Geometry check sheet. Reference: the model listing, model coordinates, mm. A direction names the side the tool comes from. Coordinates: 2 decimals unless noted, no trailing zeros. Write each loop counter-clockwise with the first axis right and the second up, starting at its lowest first coordinate (ties: lowest second). Pieces come first, ordered by that corner, then holes. Notation, with made-up numbers: (25, 51) -> (63, 51) arc R19 cw to (63, 61) -> close; hole circle Ø6 at (-5.75, -10). An arc over 180 degrees is marked (long way). Answer in a Markdown table with one row per item. Add a question column.
Q1. Thickness scan on line 1 (Y direction, x = 5, z = 1.7); line 2 (X direction, y = 10.5, z = 3); line 3 (Y direction, x = 5.5, z = 2.6). Record the ranges inside material, lowest first.
Q2. Section check A-A, the plane y = 10.5. Record the boundary of the cut face in (x, z), and give its area (3 significant figures).
Q3. Gauge pin test, flat ends, axial feed: P1, Ø1.2, axis at y = 7.5, z = 2, coming from the +X side; P2, Ø1.2, axis at x = -3, z = 2, coming from the -Y side. Record the tip position at first contact, or that the pin passes through.
Q4. Section check B-B, the plane x = 5. Record the boundary of the cut face in (y, z), and give its area (3 significant figures).
Q5. Release check for a two-part mould opening along Y. For faces 4 (the face through (5.211, 26.598, 1.972)), 5 (the face through (4.583, 24.094, 1.972)), 6 (the face through (7, 13.5, 4)) record: pulls with the +Y half, pulls with the -Y half, needs draft (parallel to the pull), parting line crosses it, or undercut.
Q6. Tool access check on faces 1 (the face through (0, 6, 2)), 2 (the face through (12, 12, 2)), 3 (the face through (-4.6, 15, 2)). Record the directions out of +Z, -Z, +X, -X, +Y, -Y that give a thin tool (end or side, any length) a straight path to the whole face; none if there is none.
Q7. Section check C-C, the plane z = 1.05. Record the boundary of the cut face in (x, y).
Q8. Section check D-D, the plane y = 6. Record the boundary of the cut face in (x, z).
```python
from build123d import *

# Parameters (mm, degrees)
BOSS_EXTRUDE1_DEPTH = 4
SKETCH2_W           = 2.5
SKETCH2_H           = 4
CUT_EXTRUDE1_DEPTH  = 4
SKETCH3_R           = 3.2
CUT_EXTRUDE2_DEPTH  = 5


with BuildPart() as part:
    # Sketch1 → Boss-Extrude1 (new body)
    with BuildSketch(Plane.XY):
        with BuildLine():
            Line((0, 0), (10, 0))
            Line((10, 0), (10, 4))
            Line((10, 4), (12.5, 4))
            Line((12.5, 4), (12.5, 8))
            Line((12.5, 8), (10, 8))
            Line((10, 8), (10, 12))
            Line((10, 12), (14.6, 12))
            Line((14.6, 12), (14.6, 17))
            ThreePointArc((14.6, 17), (5, 26.6), (-4.6, 17))
            Line((-4.6, 17), (-4.6, 12))
            Line((-4.6, 12), (0, 12))
            Line((0, 12), (0, 8))
            Line((0, 8), (-2.5, 8))
            Line((-2.5, 8), (-2.5, 4))
            Line((-2.5, 4), (0, 4))
            Line((0, 4), (0, 0))
        make_face()
    extrude(amount=BOSS_EXTRUDE1_DEPTH)

    # Sketch2 → Cut-Extrude1 (cut)
    with BuildSketch(Plane.XY.offset(4)):
        with Locations((-1.25, 6)):
            Rectangle(SKETCH2_W, SKETCH2_H)
        with Locations((11.25, 6)):
            Rectangle(SKETCH2_W, SKETCH2_H)
    extrude(amount=-CUT_EXTRUDE1_DEPTH, mode=Mode.SUBTRACT)

    # Sketch3 → Cut-Extrude2 (cut, through all)
    with BuildSketch(Plane.XY):
        with Locations((5, 20.921172359)):
            Circle(SKETCH3_R)
        with Locations((5, 10.5)):
            Circle(SKETCH3_R)
    extrude(amount=CUT_EXTRUDE2_DEPTH, mode=Mode.SUBTRACT)


solid = part.part
```
Calculated:
| question | item | result |
|---|---|---|
| 1 | line 1 | y = 0 to 7.3, 13.7 to 17.72, 24.12 to 26.6 |
| 1 | line 2 | x = 0 to 1.8, 8.2 to 10 |
| 1 | line 3 | y = 0 to 7.34, 13.66 to 17.76, 24.08 to 26.59 |
| 2 | outline | (0, 0) -> (1.8, 0) -> (1.8, 4) -> (0, 4) -> close; (8.2, 0) -> (10, 0) -> (10, 4) -> (8.2, 4) -> close |
| 2 | area | 14.4 mm² |
| 3 | P1 | stops at x = 10 |
| 3 | P2 | stops at y = 12 |
| 4 | outline | (0, 0) -> (7.3, 0) -> (7.3, 4) -> (0, 4) -> close; (13.7, 0) -> (17.72, 0) -> (17.72, 4) -> (13.7, 4) -> close; (24.12, 0) -> (26.6, 0) -> (26.6, 4) -> (24.12, 4) -> close |
| 4 | area | 55.2 mm² |
| 5 | face 4 | pulls with the +Y half |
| 5 | face 5 | undercut |
| 5 | face 6 | needs draft |
| 6 | face 1 | +Z, -Z, -X, -Y |
| 6 | face 2 | +Z, -Z, +X, -Y |
| 6 | face 3 | +Z, -Z, -X, +Y, -Y |
| 7 | outline | (-4.6, 12) -> (0, 12) -> (0, 0) -> (10, 0) -> (10, 12) -> (14.6, 12) -> (14.6, 17) arc R9.6 ccw to (-4.6, 17) -> close; hole circle Ø6.4 at (5, 10.5); hole circle Ø6.4 at (5, 20.92) |
| 8 | outline | (0, 0) -> (10, 0) -> (10, 4) -> (0, 4) -> close |
